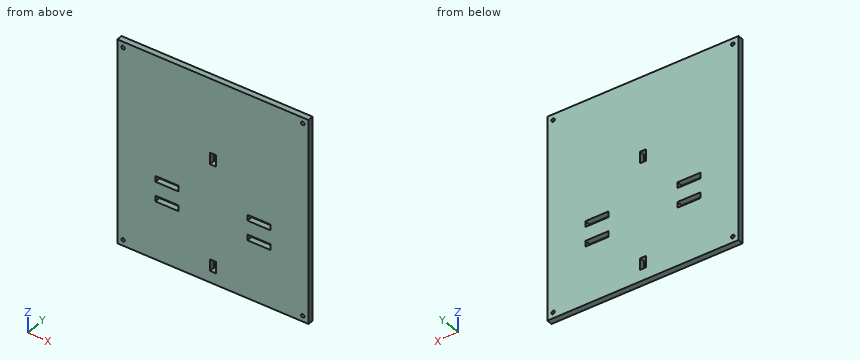
```python
from build123d import *

# Parameters (mm, degrees)
SKETCH_1_R      = 1.5
SKETCH_1_W      = 5
SKETCH_1_H      = 10
SKETCH_1_W_2    = 20
SKETCH_1_H_2    = 5
EXTRUDE_1_DEPTH = 5


with BuildPart() as part:
    # 草图1 → 凸台-拉伸1 (new body)
    with BuildSketch(Plane(origin=(0, 0, 0), x_dir=(1, 0, 0), z_dir=(0, 1, 0))):
        Polygon((0, 0), (0, 116), (0, 130.522242689), (166, 130.522242689), (166, 116), (166, 0), (166, -45.477757311), (0, -45.477757311), align=None)
        with Locations(Location((5, 125.522242689, 0), (0, 0, 270))):
            Circle(SKETCH_1_R, mode=Mode.SUBTRACT)
        with Locations(Location((161, 125.522242689, 0), (0, 0, 270))):
            Circle(SKETCH_1_R, mode=Mode.SUBTRACT)
        with Locations(Location((5, -40.477757311, 0), (0, 0, 270))):
            Circle(SKETCH_1_R, mode=Mode.SUBTRACT)
        with Locations(Location((161, -40.477757311, 0), (0, 0, 270))):
            Circle(SKETCH_1_R, mode=Mode.SUBTRACT)
        with Locations((83, 115.522242689)):
            Rectangle(SKETCH_1_W, SKETCH_1_H, mode=Mode.SUBTRACT)
        with Locations((43, 78.022242689)):
            Rectangle(SKETCH_1_W_2, SKETCH_1_H_2, mode=Mode.SUBTRACT)
        with Locations((43, 61.022242689)):
            Rectangle(SKETCH_1_W_2, SKETCH_1_H_2, mode=Mode.SUBTRACT)
        with Locations((123, 78.022242689)):
            Rectangle(SKETCH_1_W_2, SKETCH_1_H_2, mode=Mode.SUBTRACT)
        with Locations((123, 61.022242689)):
            Rectangle(SKETCH_1_W_2, SKETCH_1_H_2, mode=Mode.SUBTRACT)
        with Locations((83, 23.522242689)):
            Rectangle(SKETCH_1_W, SKETCH_1_H, mode=Mode.SUBTRACT)
    extrude(amount=EXTRUDE_1_DEPTH)


solid = part.part
```
Input: part model. Units: mm. Frame: model coordinates. Round coordinates to 2 decimals unless told otherwise and drop trailing zeros. Loops run counter-clockwise (first coordinate to the right, second up) from the corner with the lowest first, then second, coordinate; pieces in that order, holes last. Notation, with made-up numbers: (66.25, 6) - (110.25, 6) arc R12 cw to (110.25, 19) - close; hole circle Ø7 at (62, -21.75). An arc over 180 degrees is marked (long way). One line per item, written item: value. Start each with the question number.
(1) Section B-B, the plane z = -25. Return loops of the section in (x, y), plus the area to 3 significant figures.
(2) Section A-A, the plane x = 125.5. Return loops of the section in (y, z).
(3) Ray query, line 1 (Z direction, x = 161, y = 1.5); line 2 (X direction, y = 2.85, z = -22.5). Return the intervals inside material, ascending. Write a range as [from, to].
(4) Section C-C, the plane y = 3.05. Count the separate pieces of the cut face and the enclosed holes in it, plus the area to 3 significant figures.
Results below:
1. outline: (0, 0) - (80.5, 0) - (80.5, 5) - (0, 5) - close; (85.5, 0) - (166, 0) - (166, 5) - (85.5, 5) - close
1. area: 805 mm^2
2. outline: (0, -130.52) - (5, -130.52) - (5, -80.52) - (0, -80.52) - close; (0, -75.52) - (5, -75.52) - (5, -63.52) - (0, -63.52) - close; (0, -58.52) - (5, -58.52) - (5, 45.48) - (0, 45.48) - close
3. line 1: [-130.52, -127.02], [-124.02, 38.98], [41.98, 45.48]
3. line 2: [0, 80.5], [85.5, 166]
4. separate pieces: 1
4. enclosed holes: 10
4. area: 28,700 mm^2
